```python
from build123d import *

# Parameters (mm, degrees)
SKETCH1_W           = 30
SKETCH1_H           = 5
BOSS_EXTRUDE1_DEPTH = 5
SKETCH3_OUTSIDE_W   = 121.122
SKETCH3_OUTSIDE_H   = 106.762
CUT_EXTRUDE1_DEPTH  = 10
SKETCH4_R           = 1.816989411
SKETCH4_W           = 8.5
SKETCH4_H           = 5
SKETCH4_R_2         = 2.5
BOSS_EXTRUDE2_DEPTH = 5


with BuildPart() as part:
    # Sketch1 → Boss-Extrude1 (new body)
    with BuildSketch(Plane.XY):
        with Locations((15, 2.5)):
            Rectangle(SKETCH1_W, SKETCH1_H)
        with BuildLine():
            add(Edge.make_bspline(
                [(94.36042114, 75), (53.195461928, 48.027295895), (30, 5)],
                knots=[0, 0, 0, 1, 1, 1], degree=2))
            Line((30, 5), (0, 5))
            add(Edge.make_bspline(
                [(64.36042114, 75), (22.658434304, 48.707086793), (0, 5)],
                knots=[0, 0, 0, 1, 1, 1], degree=2))
            Line((64.36042114, 75), (94.36042114, 75))
        make_face()
        with Locations((79.36042114, 77.5)):
            Rectangle(SKETCH1_W, SKETCH1_H)
    extrude(amount=BOSS_EXTRUDE1_DEPTH)

    # Sketch3 outside → Cut-Extrude1 (cut)
    with BuildSketch(Plane.XY.offset(5)):
        with Locations((47.18, 40)):
            Rectangle(SKETCH3_OUTSIDE_W, SKETCH3_OUTSIDE_H)
        with BuildLine():
            Line((72.86042114, 76.5), (72.86042114, 80))
            Line((72.86042114, 80), (64.36042114, 80))
            Line((64.36042114, 80), (64.36042114, 75))
            add(Edge.make_bspline(
                [(64.36042114, 75), (22.658434304, 48.707086793), (0, 5)],
                knots=[0, 0, 0, 1, 1, 1], degree=2))
            Line((0, 5), (0, 0))
            Line((0, 0), (13.5, 0))
            Line((13.5, 0), (13.5, 3.5))
            Line((13.5, 3.5), (12, 3.5))
            ThreePointArc((12, 3.5), (10.5, 5), (12, 6.5))
            Line((12, 6.5), (13.5, 6.5))
            Line((13.5, 6.5), (13.5, 12))
            Line((13.5, 12), (16.5, 12))
            Line((16.5, 12), (16.5, 6.5))
            Line((16.5, 6.5), (18, 6.5))
            ThreePointArc((18, 6.5), (19.5, 5), (18, 3.5))
            Line((18, 3.5), (16.5, 3.5))
            Line((16.5, 3.5), (16.5, 0))
            Line((16.5, 0), (30, 0))
            Line((30, 0), (30, 5))
            add(Edge.make_bspline(
                [(30, 5), (53.195461928, 48.027295895), (94.36042114, 75)],
                knots=[0, 0, 0, 1, 1, 1], degree=2))
            Line((94.36042114, 75), (94.36042114, 80))
            Line((94.36042114, 80), (75.86042114, 80))
            Line((75.86042114, 80), (75.86042114, 76.5))
            Line((75.86042114, 76.5), (76.86042114, 76.5))
            ThreePointArc((76.86042114, 76.5), (78.36042114, 75), (76.86042114, 73.5))
            Line((76.86042114, 73.5), (75.86042114, 73.5))
            Line((75.86042114, 73.5), (75.86042114, 68))
            Line((75.86042114, 68), (72.86042114, 68))
            Line((72.86042114, 68), (72.86042114, 73.5))
            Line((72.86042114, 73.5), (71.86042114, 73.5))
            ThreePointArc((71.86042114, 73.5), (70.36042114, 75), (71.86042114, 76.5))
            Line((71.86042114, 76.5), (72.86042114, 76.5))
        make_face(mode=Mode.SUBTRACT)
    extrude(amount=-CUT_EXTRUDE1_DEPTH, mode=Mode.SUBTRACT)

    # Sketch4 → Boss-Extrude2 (add)
    with BuildSketch(Plane.XY.offset(5)):
        Polygon((94.285794486, 80), (94.36042114, 80), (94.36042114, 85), (80.86042114, 85), (80.86042114, 80), align=None)
        with Locations((96.177410551, 78.183010589)):
            Circle(SKETCH4_R)
        with BuildLine():
            Line((96.177410551, 80), (94.36042114, 80))
            Line((94.36042114, 80), (94.36042114, 78.183010589))
            ThreePointArc((94.36042114, 78.183010589), (94.892605017, 79.467816123), (96.177410551, 80))
        make_face()
        with BuildLine():
            ThreePointArc((97.020667914, 76.573548711), (95.23686262, 76.628398062), (94.36042114, 78.183010589))
            Line((94.36042114, 78.183010589), (94.36042114, 75))
            ThreePointArc((94.36042114, 75), (95.670266462, 75.821056521), (97.020667914, 76.573548711))
        make_face()
        with Locations((25.75, -2.5)):
            Rectangle(SKETCH4_W, SKETCH4_H)
        with Locations((4.25, -2.5)):
            Rectangle(SKETCH4_W, SKETCH4_H)
        with BuildLine():
            Line((30, 5), (30, 0))
            ThreePointArc((30, 0), (31.767766953, 0.732233047), (32.5, 2.5))
            ThreePointArc((32.5, 2.5), (31.767766953, 4.267766953), (30, 5))
        make_face()
        with BuildLine():
            ThreePointArc((30, 5), (27.5, 2.5), (30, 0))
            Line((30, 0), (30, 5))
        make_face()
        with Locations((0, 2.5)):
            Circle(SKETCH4_R_2)
    extrude(amount=-BOSS_EXTRUDE2_DEPTH)


solid = part.part
```
Input: part model. Units: mm. Frame: model coordinates. A direction names the side the tool comes from. Round coordinates to 2 decimals unless told otherwise and drop trailing zeros. One line per item, written item: value.
(1) Material intervals for line 1 (X direction, y = -0.5, z = 1.25); line 2 (X direction, y = 8, z = 4.7); line 3 (Y direction, x = 30.5, z = 2.1), sorted ascending. Write a range as [from, to].
Geometry check:
line 1: [0, 8.5], [21.5, 30]
line 2: [1.59, 13.5], [16.5, 31.65]
line 3: [0.05, 4.95], [5.92, 47.62]
(2) Mould query, pull axis X, two halves, no side actions, for faces 5 (the face through (78.36, 75.03, 2.54)), 6 (the face through (94.36, 82, 3)), 7 (the face through (4, -5, 3)), 8 (the face through (72.86, 78, 3)). Classes: pulls with the +X half, pulls with the -X half, needs draft (parallel to the pull), parting line crosses it, or undercut.
Geometry check:
face 5: undercut
face 6: pulls with the +X half
face 7: needs draft
face 8: undercut
(3) Pin query (flat end, axial travel): pin 1 (1 mm diameter, centred on y = 2.5, z = 3.5, fed in from +X); pin 2 (3 mm diameter, centred on y = 34.5, z = 1.5, fed in from +X); pin 3 (1.1 mm diameter, centred on x = 76, z = 2.5, fed in from -Y); pin 4 (3 mm diameter, centred on y = 77.5, z = 2.5, fed in from +X). Return the tip coordinate at first contact, or that it passes through.
Geometry check:
pin 1: x = 32.5
pin 2: x = 50.73
pin 3: y = 60.97
pin 4: x = 97.99
(4) Set-up query: faces 1 (the face through (80.86, 83, 3)), 2 (the face through (13.5, 2, 3)), 3 (the face through (30, -3, 3)), 4 (the face through (19.5, 5, 2.5)). Return all of +Z, -Z, +X, -X, +Y, -Y with unobstructed straight access to the full face (end or side cutting, diameter ignored); none if empty.
Geometry check:
face 1: +Z, -Z, -X, +Y
face 2: +Z, -Z, -Y
face 3: +Z, -Z, +X, -Y
face 4: +Z, -Z
